```python
from build123d import *

# Parameters (mm, degrees)
PAD_DEPTH    = 4
PAD001_DEPTH = 5
SKETCH002_W  = 40
SKETCH002_H  = 2
POCKET_DEPTH = 20


with BuildPart() as part:
    # Sketch → Pad (new body)
    with BuildSketch(Plane.XY):
        with BuildLine():
            Line((4.5, 0), (95.5, 0))
            ThreePointArc((95.5, 0), (98.681981, 1.318019), (100, 4.5))
            Line((100, 4.5), (100, 75.5))
            ThreePointArc((100, 75.5), (98.681981, 78.681981), (95.5, 80))
            Line((95.5, 80), (4.5, 80))
            ThreePointArc((4.5, 80), (1.318019, 78.681981), (0, 75.5))
            Line((0, 75.5), (0, 4.5))
            ThreePointArc((0, 4.5), (1.318019, 1.318019), (4.5, 0))
        make_face()
    extrude(amount=PAD_DEPTH)

    # Sketch001 (on Face10 of Pad) → Pad001 (join)
    with BuildSketch(Plane.XY.offset(4)):
        with BuildLine():
            Line((2.5, 74.5), (2.5, 4.5))
            ThreePointArc((2.5, 4.5), (3.085786, 3.085786), (4.5, 2.5))
            Line((4.5, 2.5), (94.5, 2.5))
            ThreePointArc((94.5, 2.5), (95.914214, 3.085786), (96.5, 4.5))
            Line((96.5, 4.5), (96.5, 74.5))
            ThreePointArc((96.5, 74.5), (95.914214, 75.914214), (94.5, 76.5))
            Line((94.5, 76.5), (4.5, 76.5))
            ThreePointArc((4.5, 76.5), (3.085786, 75.914214), (2.5, 74.5))
        make_face()
    extrude(amount=PAD001_DEPTH)

    # Sketch002 (on Face4 of Pad001) → Pocket (cut)
    with BuildSketch(Plane(origin=(0, 0, 0), x_dir=(1, 0, 0), z_dir=(0, 0, -1))):
        with Locations((50, -46)):
            Rectangle(SKETCH002_W, SKETCH002_H)
        with Locations((50, -42)):
            Rectangle(SKETCH002_W, SKETCH002_H)
        with Locations((50, -38)):
            Rectangle(SKETCH002_W, SKETCH002_H)
        with Locations((50, -34)):
            Rectangle(SKETCH002_W, SKETCH002_H)
        with Locations((50, -30)):
            Rectangle(SKETCH002_W, SKETCH002_H)
        with Locations((50, -26)):
            Rectangle(SKETCH002_W, SKETCH002_H)
    extrude(amount=-POCKET_DEPTH, mode=Mode.SUBTRACT)


solid = part.part
```
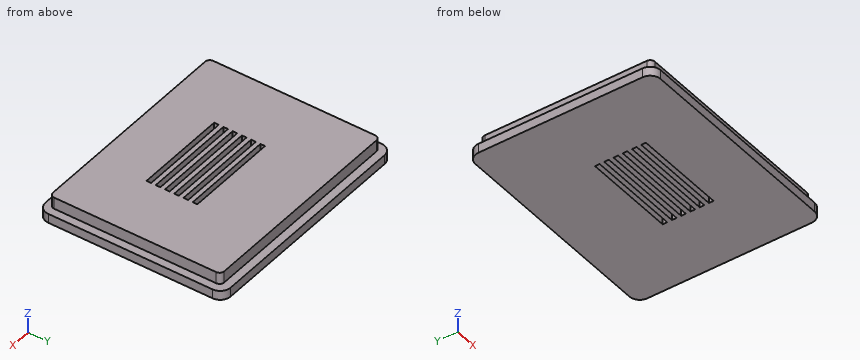
Work out the finished part from the listing and answer in its coordinate system (mm). Give positions to 0.01 mm unless a question says otherwise; leave off trailing zeros. Loops run counter-clockwise (first coordinate to the right, second up) from the corner with the lowest first, then second, coordinate; pieces in that order, holes last. Notation, with made-up numbers: (51, -8) -> (91, -8) arc R14 ccw to (91, 6) -> close; hole circle Ø9 at (15, 52.5). An arc over 180 degrees is marked (long way). Write item = value, one per line. Start each with the question number.
(1) Find section D-D on x = 27. Give the vertices of the cut face in (y, z).
(2) Given pin 1 Ø5 at (x, y) = (56.5, 11.5) entering from -Z; pin 2 Ø1.5 at (x, z) = (41, 5.5) entering from -Y; pin 3 Ø2 at (y, z) = (70.5, 7) entering from -X; pin 4 Ø1 at (y, z) = (46, 5.5) entering from +X, each flat-ended and moving along its own axis, determine where each tip first touches the part or whether it passes through.
(3) Find section C-C on y = 60.5. Give the vertices of the cut face in (x, z), and give its area (3 significant figures).
(4) Find section A-A on z = 1.75. Give the number of separate pieces and of enclosed holes in the cut face, and give its area (3 significant figures).
(5) Find the intervals of material crossed by probe 1 along X at (y, z) = (30.5, 6.5); probe 2 along X at (y, z) = (26, 0.5); probe 3 along X at (y, z) = (16, 4.25), in increasing order. Write a range as from..to.
From the geometry:
q1.outline = (0, 0) -> (80, 0) -> (80, 4) -> (76.5, 4) -> (76.5, 9) -> (2.5, 9) -> (2.5, 4) -> (0, 4) -> close
q2.pin_1 = 0
q2.pin_2 = 2.5
q2.pin_3 = 2.5
q2.pin_4 = 96.5
q3.outline = (0, 0) -> (100, 0) -> (100, 4) -> (96.5, 4) -> (96.5, 9) -> (2.5, 9) -> (2.5, 4) -> (0, 4) -> close
q3.area = 870 mm^2
q4.separate_pieces = 1
q4.enclosed_holes = 6
q4.area = 7,500 mm^2
q5.probe_1 = 2.5..30, 70..96.5
q5.probe_2 = 0..30, 70..100
q5.probe_3 = 2.5..96.5
